Can you work these out from the drawing? Everything is in mm from the part's minimum corner. A direction names the side the tool comes from. Coordinates: 2 decimals unless noted, no trailing zeros. Write each loop counter-clockwise with the first axis right and the second up, starting at its lowest first coordinate (ties: lowest second). Pieces come first, ordered by that corner, then holes.
(1) Thinking about a two-plate mould opening in Y: for the marked faces 1, 2 and 3, which applies, released by +Y, released by -Y, zero draft, split by the parting line, or undercut?
(2) Please list where these lines run through material, in increasing order: probe 1 along X at (y, z) = (67.5, 34); probe 2 along Z at (x, y) = (25.5, 26.5).
(3) For pin 1 Ø20.5 at (x, y) = (15, 69) entering from +Z; pin 2 Ø12.5 at (x, z) = (60.5, 47) entering from -Y; pin 3 Ø4 at (x, y) = (33.5, 62) entering from +Z; pin 4 Ø12.5 at (x, z) = (16, 24) entering from -Y, each with a flat end and sliding along its axis, tell me the tip position at first contact or that it passes through.
(4) Imagine slicing it at C-C, the plane x = 58. List the corners of the cut face in (y, z) for me, plus the area to 3 significant figures.
(5) Which directions (+Z, -Z, +X, -X, +Y, -Y) give clear straight access to the entire face, cutting with the end or side of a thin tool? Please do the marked faces 4, 5, 6 and 7.
(6) Imagine slicing it at D-D, the plane z = 22.5. List the corners of the cut face in (x, y) for me.
(7) Imagine slicing it at B-B, the plane y = 12. List the corners of the cut face in (x, z) for me, plus the area to 3 significant figures.
(8) Imagine slicing it at A-A, the plane z = 33.5. List the corners of the cut face in (x, y) for me, plus the area to 3 significant figures.
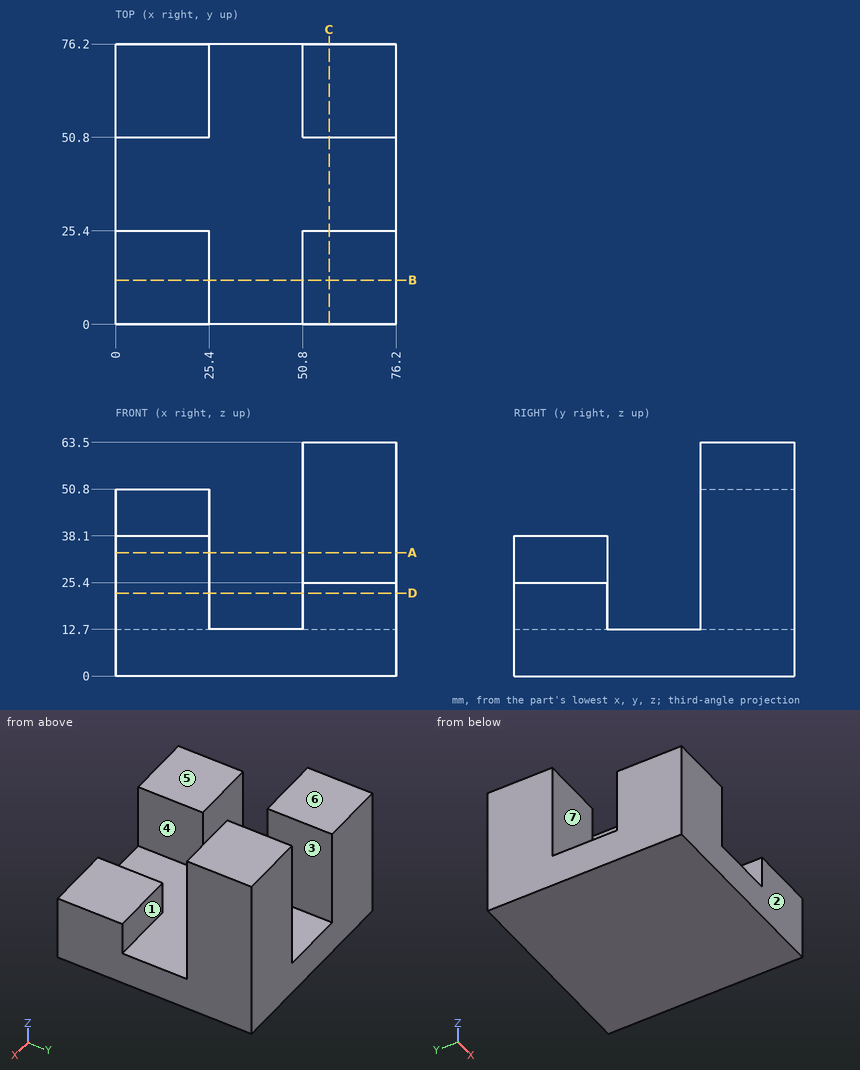
Recorded:
1. face 1: undercut
1. face 2: released by -Y
1. face 3: zero draft
2. probe 1: x = 0 to 25.4, 50.8 to 76.2
2. probe 2: z = 0 to 12.7
3. pin 1: stops at z = 50.8
3. pin 2: stops at y = 50.8
3. pin 3: stops at z = 12.7
3. pin 4: stops at y = 0
4. outline: (0, 0) - (76.2, 0) - (76.2, 63.5) - (50.8, 63.5) - (50.8, 12.7) - (25.4, 12.7) - (25.4, 25.4) - (0, 25.4) - close
4. area: 2,580 mm2
5. face 4: +Z, +Y, -Y
5. face 5: +Z, +X, -X, -Y
5. face 6: +Z, -X, +Y, -Y
5. face 7: +Z, +X, -X
6. outline: (0, 0) - (25.4, 0) - (25.4, 25.4) - (0, 25.4) - close; (0, 50.8) - (25.4, 50.8) - (25.4, 76.2) - (0, 76.2) - close; (50.8, 0) - (76.2, 0) - (76.2, 25.4) - (50.8, 25.4) - close; (50.8, 50.8) - (76.2, 50.8) - (76.2, 76.2) - (50.8, 76.2) - close
7. outline: (0, 0) - (76.2, 0) - (76.2, 25.4) - (50.8, 25.4) - (50.8, 12.7) - (25.4, 12.7) - (25.4, 38.1) - (0, 38.1) - close
7. area: 1,940 mm2
8. outline: (0, 0) - (25.4, 0) - (25.4, 25.4) - (0, 25.4) - close; (0, 50.8) - (25.4, 50.8) - (25.4, 76.2) - (0, 76.2) - close; (50.8, 50.8) - (76.2, 50.8) - (76.2, 76.2) - (50.8, 76.2) - close
8. area: 1,940 mm2
